Geometry: final body of the model. Coordinates: model frame, mm. A direction names the side the tool comes from. Round coordinates to 2 decimals unless told otherwise and drop trailing zeros. Loops run counter-clockwise (first coordinate to the right, second up) from the corner with the lowest first, then second, coordinate; pieces in that order, holes last. Notation, with made-up numbers: M 24.5,74.25 L 28.5,74.25 A20 ccw 28.5,104.25 Z; hole C -26.75,27 d3. An arc over 180 degrees is marked long. Answer as a JSON object with one key per item and string values.
from build123d import *
from build123d.topology import SkipClean

# Parameters (mm, degrees)
SKETCH1_R           = 1.15
BOSS_EXTRUDE1_DEPTH = 8
BOSS_EXTRUDE2_START = 13
SKETCH4_R           = 8
SKETCH4_R_2         = 1.15
BOSS_EXTRUDE2_DEPTH = 13
CUT_EXTRUDE3_DEPTH  = 15.5
CUT_EXTRUDE4_DEPTH  = 5.5
BOSS_EXTRUDE3_START = -13
BOSS_EXTRUDE3_DEPTH = 13


with BuildPart() as part:
    # Sketch1 → Boss-Extrude1 (new body)
    with BuildSketch(Plane.XY):
        with BuildLine():
            Line((0, -42), (0, -40))
            ThreePointArc((0, -40), (22.793187837, -20.077432085), (6.099520657, 5.176470588))
            ThreePointArc((6.099520657, 5.176470588), (7.259881704, -3.360672202), (0, -8))
            ThreePointArc((0, -8), (-8, 0), (0, 8))
            ThreePointArc((0, 8), (25, -17), (0, -42))
        make_face()
        with Locations((0, 6)):
            Circle(SKETCH1_R, mode=Mode.SUBTRACT)
        with Locations((-6, 0)):
            Circle(SKETCH1_R, mode=Mode.SUBTRACT)
        with Locations((0, -6)):
            Circle(SKETCH1_R, mode=Mode.SUBTRACT)
        with Locations((6, 0)):
            Circle(SKETCH1_R, mode=Mode.SUBTRACT)
    extrude(amount=BOSS_EXTRUDE1_DEPTH)

    # Sketch4 → Boss-Extrude2 (add)
    with SkipClean():  # the faces are left unmerged after this step: merging them gives an invalid solid
        with BuildSketch(Plane(origin=(0, 0, 0), x_dir=(-1, 0, 0), z_dir=(0, 0, -1)).offset(BOSS_EXTRUDE2_START)):
            Circle(SKETCH4_R)
            with Locations((0, 6)):
                Circle(SKETCH4_R_2, mode=Mode.SUBTRACT)
            with Locations((-6, 0)):
                Circle(SKETCH4_R_2, mode=Mode.SUBTRACT)
            with Locations((0, -6)):
                Circle(SKETCH4_R_2, mode=Mode.SUBTRACT)
            with Locations((6, 0)):
                Circle(SKETCH4_R_2, mode=Mode.SUBTRACT)
        extrude(amount=-BOSS_EXTRUDE2_DEPTH)

    # Sketch3 → Cut-Extrude3 (cut)
    with BuildSketch(Plane.XY.offset(8)):
        with BuildLine():
            Line((6, 2), (10, 2))
            Line((10, 2), (10, -2))
            Line((10, -2), (6, -2))
            ThreePointArc((6, -2), (4, 0), (6, 2))
        make_face()
        with BuildLine():
            Line((2, -6), (2, -10))
            Line((2, -10), (-2, -10))
            Line((-2, -10), (-2, -6))
            ThreePointArc((-2, -6), (0, -4), (2, -6))
        make_face()
        with BuildLine():
            Line((-6, -2), (-10, -2))
            Line((-10, -2), (-10, 2))
            Line((-10, 2), (-6, 2))
            ThreePointArc((-6, 2), (-4, 0), (-6, -2))
        make_face()
        with BuildLine():
            Line((-2, 6), (-2, 10))
            Line((-2, 10), (2, 10))
            Line((2, 10), (2, 6))
            ThreePointArc((2, 6), (0, 4), (-2, 6))
        make_face()
    extrude(amount=-CUT_EXTRUDE3_DEPTH, mode=Mode.SUBTRACT)

    # Sketch5 → Cut-Extrude4 (cut)
    with BuildSketch(Plane(origin=(0, 0, -13), x_dir=(-1, 0, 0), z_dir=(0, 0, -1))):
        with BuildLine():
            Line((-3.420800345, 1.975), (-6.92820323, 4))
            ThreePointArc((-6.92820323, 4), (2.070552361, -7.72740661), (4, 6.92820323))
            Line((4, 6.92820323), (1.975, 3.420800345))
            ThreePointArc((1.975, 3.420800345), (3.821665179, 0.998686766), (3.396076023, -2.017217799))
            Line((3.396076023, -2.017217799), (4.103182804, -2.72432458))
            Line((4.103182804, -2.72432458), (2.72432458, -4.103182804))
            Line((2.72432458, -4.103182804), (2.017217799, -3.396076023))
            ThreePointArc((2.017217799, -3.396076023), (-2.775720699, -2.810315747), (-3.420800345, 1.975))
        make_face()
    extrude(amount=-CUT_EXTRUDE4_DEPTH, mode=Mode.SUBTRACT)

    # Sketch6 → Boss-Extrude3 (add)
    with BuildSketch(Plane.XY.offset(8).offset(BOSS_EXTRUDE3_START)):
        with BuildLine():
            Line((5.656854249, 5.656854249), (0, 0))
            Line((0, 0), (-5.656854249, 5.656854249))
            ThreePointArc((-5.656854249, 5.656854249), (0, -8), (5.656854249, 5.656854249))
        make_face()
    extrude(amount=BOSS_EXTRUDE3_DEPTH)


with BuildPart() as body_2:
    # Mirror2: mirrored copy
    add(part.part.mirror(Plane.XY))


solid = body_2.part
1) Reachability of faces 1 (the flat face through (-2, 7, 0)), 2 (the flat face through (-4, -1, 7.5)), 3 (the cylindrical face through (4, 0, 6)) from +Z, -Z, +X, -X, +Y, -Y: full face, straight path, thin tool, end or side. Return the list, or none.
Results:
{"face 1": "-Z, +Y", "face 2": "+Z", "face 3": "+Z, +X"}
2) Section query C-C (z = 11). Return the cut outline in (x, y) (3 decimals), and give its area (3 significant figures).
Results:
{"outline": "M -4.103,-2.724 L -2.724,-4.103 L -2.017,-3.396 A3.95 ccw 3.421,1.975 L 6.928,4 A8 ccw -4,6.928 L -1.975,3.421 A3.95 ccw -3.396,-2.017 Z; hole C 0,6 d2.3", "area": "84.7 mm2"}
3) Pull-direction query (X, two-part tool) for faces 4 (the flat face through (0, 2, 13)), 5 (the flat face through (2, 7, 0)), 6 (the cylindrical face through (-3.81, 1.04, 10.29)); classes: +X half, -X half, draft (parallel to the pull), parting line (faces both ways), or undercut.
Results:
{"face 4": "draft", "face 5": "undercut", "face 6": "-X half"}
4) Section query D-D (y = -17). Return the cut outline in (x, z), and give its area (3 significant figures).
Results:
{"outline": "M 23,-8 L 25,-8 L 25,0 L 23,0 Z", "area": "16.0 mm2"}
5) Pin query (flat end, axial travel): P1, Ø0.5, axis at y = -7, z = 6, coming from the +X side; P2, Ø5, axis at x = 5, z = 9.5, coming from the +Y side; P3, Ø1, axis at x = -2.5, z = 8.5, coming from the -Y side; P4, Ø8, axis at x = 4, z = 8, coming from the +Y side. Return the tip coordinate at first contact, or that it passes through.
Results:
{"P1": "x = 4.29", "P2": "y = 7.6", "P3": "y = -4.1", "P4": "y = 8"}
6) Ray query, line 1 (Y direction, x = 0, z = 10.05); line 2 (Z direction, x = 10, y = -39.5); line 3 (Z direction, x = -7, y = 0). Return the intervals inside material, ascending.
Results:
{"line 1": "-3.95 to 4.85, 7.15 to 8", "line 2": "-8 to 0", "line 3": "-8 to 5"}
7) Section query B-B (z = 5.75). Return the cut outline in (x, y).
Results:
{"outline": "M -7.75,-2 A8 ccw -2,-7.75 L -2,-6 A2 cw 2,-6 L 2,-7.75 A8 ccw 7.75,-2 L 6,-2 A2 cw 6,2 L 7.75,2 A8 ccw 2,7.75 L 2,6 A2 cw -2,6 L -2,7.75 A8 ccw -7.75,2 L -6,2 A2 cw -6,-2 Z"}
8) Section query A-A (x = 21.5). Return the cut outline in (y, z).
Results:
{"outline": "M -29.76,-8 L -25.17,-8 L -25.17,0 L -29.76,0 Z; M -8.83,-8 L -4.24,-8 L -4.24,0 L -8.83,0 Z"}
